The drawing under review shows one solid part. Ordinate dimensions are in mm from its lowest x, y, z. A direction names the side the tool comes from. Round coordinates to 2 decimals unless told otherwise and drop trailing zeros. Order: outer loops, then holes, each group sorted by start corner. A loop starts at its lowest first (then second) coordinate and runs counter-clockwise, first axis right, second up. Notation, with made-up numbers: M 49,51 L 107,51 A22 ccw 107,66 Z; hole C 88,48.25 d7. An arc over 180 degrees is marked long. Use a Markdown table: item, result.
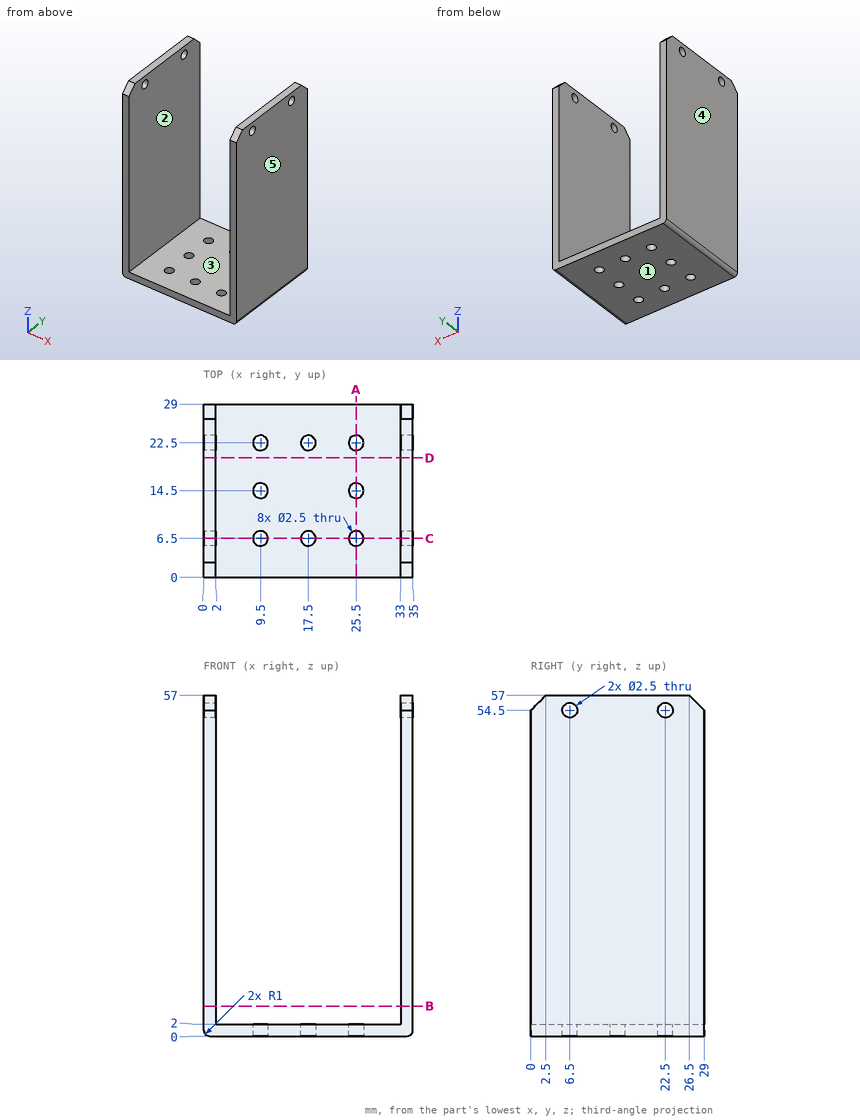
Q1. Wall thickness on line 1 along Y through (x, z) = (25.5, 0.6); line 2 along X through (y, z) = (3.5, 7); line 3 along Z through (x, y) = (7.5, 2.5): over which ranges is each line inside the solid? List them lowest first. Write a range as [from, to].
Determined:
| item | result |
|---|---|
| line 1 | y = [0, 5.25], [7.75, 13.25], [15.75, 21.25], [23.75, 29] |
| line 2 | x = [0, 2], [33, 35] |
| line 3 | z = [0, 2] |
Q2. Add section D-D (y = 20). Write out the cut boundary in (x, z).
Determined:
| item | result |
|---|---|
| outline | M 0,1 A1 ccw 1,0 L 34,0 A1 ccw 35,1 L 35,57 L 33,57 L 33,2 L 2,2 L 2,57 L 0,57 Z |
Q3. Add section A-A (x = 25.5). Write out the cut boundary in (y, z).
Determined:
| item | result |
|---|---|
| outline | M 0,0 L 5.25,0 L 5.25,2 L 0,2 Z; M 7.75,0 L 13.25,0 L 13.25,2 L 7.75,2 Z; M 15.75,0 L 21.25,0 L 21.25,2 L 15.75,2 Z; M 23.75,0 L 29,0 L 29,2 L 23.75,2 Z |
Q4. Add section B-B (z = 5). Write out the cut boundary in (x, y), then the cut area to 3 significant figures.
Determined:
| item | result |
|---|---|
| outline | M 0,0 L 2,0 L 2,29 L 0,29 Z; M 33,0 L 35,0 L 35,29 L 33,29 Z |
| area | 116 mm^2 |
Q5. Add section C-C (y = 6.5). Give the number of separate pieces and of enclosed holes in the cut face, then the cut area to 3 significant figures.
Determined:
| item | result |
|---|---|
| separate pieces | 6 |
| enclosed holes | 0 |
| area | 265 mm^2 |
Q6. Machinability: for the marked faces 1 and 2, which of the approach directions +Z, -Z, +X, -X, +Y, -Y give a long, thin tool a straight path to every point of the face, cutting with its end or side? Answer none if there is none.
Determined:
| item | result |
|---|---|
| face 1 | -Z, +X, -X, +Y, -Y |
| face 2 | +Z, +Y, -Y |
Q7. Clearance check with flat-ended pins moving along their axes: pin 1 (6 mm diameter, centred on x = 19.5, y = 14, fed in from +Z); pin 2 (3 mm diameter, centred on y = 22.5, z = 54.5, fed in from -X). State where each tip first meets the part, or that it passes through.
Determined:
| item | result |
|---|---|
| pin 1 | stops at z = 2 |
| pin 2 | stops at x = 0 |
Q8. Draft analysis for pull direction X (two halves, no side actions). For the marked faces 3, 4 and 5, state which applies: pulls with the +X half, pulls with the -X half, needs draft (parallel to the pull), parting line crosses it, or undercut.
Determined:
| item | result |
|---|---|
| face 3 | undercut |
| face 4 | pulls with the -X half |
| face 5 | pulls with the +X half |
